Design review of the part built by this model. Coordinates are the model's own, in mm. A direction names the side the tool comes from. Coordinates: 2 decimals unless noted, no trailing zeros. Loops run counter-clockwise (first coordinate to the right, second up) from the corner with the lowest first, then second, coordinate; pieces in that order, holes last.
from build123d import *

# Parameters (mm, degrees)
SKETCH1_R               = 1.65
BOSS_EXTRUDE1_DEPTH     = 11.7
CUT_EXTRUDE1_DEPTH      = 51
CUT_EXTRUDE1_DEPTH_BACK = 10
FILLET1_R               = 3
FILLET2_R               = 5
SKETCH3_R               = 3
CUT_EXTRUDE2_DEPTH      = 5.7


with BuildPart() as part:
    # Sketch1 → Boss-Extrude1 (new body)
    with BuildSketch(Plane(origin=(0, 0, 0), x_dir=(1, 0, 0), z_dir=(0, 1, 0))):
        Polygon((-22.5, 37), (22.5, 37), (53, 0), (75, 0), (75, 12.409836066), (30, 67), (-30, 67), (-75, 12.409836066), (-75, 0), (-53, 0), align=None)
        with Locations(Location((70.5, 5, 0), (0, 0, 270))):
            Circle(SKETCH1_R, mode=Mode.SUBTRACT)
        with Locations(Location((-70.5, 5, 0), (0, 0, 270))):
            Circle(SKETCH1_R, mode=Mode.SUBTRACT)
    extrude(amount=BOSS_EXTRUDE1_DEPTH)

    # Sketch2 → Cut-Extrude1 (cut, two sides: drawn at the far end of the back side and taken through both)
    with BuildSketch(Plane(origin=(0, 0, 0), x_dir=(1, 0, 0), z_dir=(0, 1, 0)).offset(-CUT_EXTRUDE1_DEPTH_BACK)):
        Polygon((-65, 15.108099284), (-65, 0), (-53, 0), (-22.5, 37), (0, 37), (0, 62), (-26.345865626, 62), align=None)
        Polygon((26.345865626, 62), (0, 62), (0, 37), (22.5, 37), (53, 0), (65, 0), (65, 15.108099284), align=None)
    extrude(amount=CUT_EXTRUDE1_DEPTH + CUT_EXTRUDE1_DEPTH_BACK, mode=Mode.SUBTRACT)

    # Fillet1
    fillet1_edges = [part.edges().sort_by_distance(p)[0] for p in [
        (52.5, 11.7, -39.704918033),
        (0, 11.7, -67),
        (-52.5, 11.7, -39.704918033),
    ]]
    fillet(fillet1_edges, radius=FILLET1_R)

    # Fillet2
    # the kernel refuses this fillet: 5 mm, written as the material it takes off along each edge
    with BuildSketch(Plane(origin=(27.641824959, 11.7, -62), x_dir=(0.7716291513697928, 0, -0.6360726788318559), z_dir=(0.6360726788318559, 0, 0.7716291513697928))) as fillet2_piece_1:
        with BuildLine():
            CenterArc((2, -3), 3, 0, 90)
            Line((5, -3), (5, 0))
            Line((5, 0), (2, 0))
        make_face()
    revolve(axis=Axis((27.641824959, 11.7, -62), (0, 1, 0)), revolution_arc=50.50041147, mode=Mode.SUBTRACT)
    with BuildSketch(Plane(origin=(-27.641824959, 11.7, -62), x_dir=(0, 0, -1), z_dir=(1, 0, 0))) as fillet2_piece_2:
        with BuildLine():
            CenterArc((2, -3), 3, 0, 90)
            Line((5, -3), (5, 0))
            Line((5, 0), (2, 0))
        make_face()
    revolve(axis=Axis((-27.641824959, 11.7, -62), (0, 1, 0)), revolution_arc=50.50041147, mode=Mode.SUBTRACT)
    with BuildSketch(Plane(origin=(-30, -5.895437603, -67), x_dir=(-0.6360726788318558, 0, 0.771629151369793), z_dir=(0, 1, 0)), Plane(origin=(30, -5.895437603, -67), x_dir=(-1, 0, 0), z_dir=(0, 1, 0))) as fillet2_piece_3:
        with BuildLine():
            CenterArc((FILLET2_R * 0.471635008245, FILLET2_R), FILLET2_R, 219.49958853, 50.50041147)
            Line((-FILLET2_R * 0.299994143125, FILLET2_R * 0.363927321168), (0, 0))
            Line((0, 0), (FILLET2_R * 0.471635008245, 0))
        make_face()
    extrude(amount=17.595437603, mode=Mode.SUBTRACT)

    # Sketch3 → Cut-Extrude2 (cut)
    with BuildSketch(Plane(origin=(0, 11.7, 0), x_dir=(1, 0, 0), z_dir=(0, 1, 0))):
        with Locations(Location((-70.5, 5, 0), (0, 0, 270))):
            Circle(SKETCH3_R)
        with Locations(Location((70.5, 5, 0), (0, 0, 270))):
            Circle(SKETCH3_R)
    extrude(amount=-CUT_EXTRUDE2_DEPTH, mode=Mode.SUBTRACT)


solid = part.part
Q1. For line 1 (X direction, y = 7.6, z = -5); line 2 (X direction, y = 3.35, z = -5); line 3 (Z direction, x = 20, y = 4), list the stretches that pass through material, from the lowest coordinate up.
Q2. Take a section at A-A, the plane z = -5. Write out the cut boundary in (x, y).
Q3. Machinability: for faces 5 (the flat face through (0, 11.7, -63)), 6 (the flat face through (-45.402, 5.768, -38.882)), 7 (the flat face through (69, 6, -4)), which of the approach directions +Z, -Z, +X, -X, +Y, -Y give a long, thin tool a straight path to every point of the face, cutting with its end or side? Answer none if there is none.
Q4. Take a section at C-C, the plane x = -19. Write out the cut boundary in (y, z), then the cut area to 3 significant figures.
Q5. The part is to be moulded in two halves that separate along Z. For faces 1 (the cylindrical face through (-54.068, 10.798, -36.458)), 2 (the flat face through (-75, 6, -6)), 3 (the flat face through (0, 6, -62)), 4 (the cylindrical face through (-72.1, 3, -5.4)), say which applies: pulls with the +Z half, pulls with the -Z half, needs draft (parallel to the pull), parting line crosses it, or undercut.
Q6. Clearance check with flat-ended pins moving along their axes: pin 1 Ø3 at (x, z) = (70.5, -5) entering from +Y; pin 2 Ø3 at (x, z) = (71.5, -5) entering from +Y; pin 3 Ø1.5 at (y, z) = (3.5, -58) entering from -X; pin 4 Ø5 at (x, y) = (4.5, 2.5) entering from +Z. State where each tip first meets the part, or that it passes through.
Q7. Take a section at B-B, the plane y = 3.75. Write out the cut boundary in (x, z).
Entries:
1. line 1: x = -75 to -73.5, -67.5 to -65, 65 to 67.5, 73.5 to 75
1. line 2: x = -75 to -72.15, -68.85 to -65, 65 to 68.85, 72.15 to 75
1. line 3: z = -67 to -62
2. outline: (-75, 0) - (-72.15, 0) - (-72.15, 6) - (-73.5, 6) - (-73.5, 11.7) - (-75, 11.7) - close; (-68.85, 0) - (-65, 0) - (-65, 11.7) - (-67.5, 11.7) - (-67.5, 6) - (-68.85, 6) - close; (65, 0) - (68.85, 0) - (68.85, 6) - (67.5, 6) - (67.5, 11.7) - (65, 11.7) - close; (72.15, 0) - (75, 0) - (75, 11.7) - (73.5, 11.7) - (73.5, 6) - (72.15, 6) - close
3. face 5: +Z, -Z, +X, -X, +Y
3. face 6: +Z, +Y, -Y
3. face 7: +Y
4. outline: (0, -67) - (8.7, -67) arc R3 ccw to (11.7, -64) - (11.7, -62) - (0, -62) - close
4. area: 56.6 mm2
5. face 1: pulls with the -Z half
5. face 2: needs draft
5. face 3: pulls with the +Z half
5. face 4: undercut
6. pin 1: passes through
6. pin 2: stops at y = 6
6. pin 3: stops at x = -38.04
6. pin 4: stops at z = -62
7. outline: (-75, -12.41) - (-31.5, -65.18) arc R5 ccw to (-27.64, -67) - (27.64, -67) arc R5 ccw to (31.5, -65.18) - (75, -12.41) - (75, 0) - (65, 0) - (65, -15.11) - (26.35, -62) - (-26.35, -62) - (-65, -15.11) - (-65, 0) - (-75, 0) - close; hole circle Ø3.3 at (-70.5, -5); hole circle Ø3.3 at (70.5, -5)
